Design review of the part built by this model. Coordinates are the model's own, in mm. A direction names the side the tool comes from. Give positions to 0.01 mm unless a question says otherwise; leave off trailing zeros. Loops run counter-clockwise (first coordinate to the right, second up) from the corner with the lowest first, then second, coordinate; pieces in that order, holes last. Notation, with made-up numbers: (43, 9) -> (69, 9) arc R12 ccw to (69, 23) -> close; hole circle Ø11 at (36.5, -8). An arc over 180 degrees is marked (long way). Use CSV: the item, a comma, the result in double quotes. Start each with the question number.
Item 1: We need section C-C (z = 0). State the section outline as (x, y) points, plus the area to 3 significant figures.
Item 2: Clearance check with flat-ended pins moving along their axes: pin 1 (0.6 mm diameter, centred on x = 16.5, z = -1.5, fed in from -Y); pin 2 (1 mm diameter, centred on x = 7.5, y = 1, fed in from -Z); pin 3 (1 mm diameter, centred on y = 1, z = -0.5, fed in from +X). State where each tip first meets the part, or that it passes through.
Item 3: We need section D-D (x = 10.75). State the section outline as (y, z) points, plus the area to 3 significant figures.
Item 4: The part is to be moulded in two halves that separate along Z. For faces 4 (the face through (16, 0, -1.677)), 5 (the face through (13.9, 0, 0)), 6 (the face through (16, 0, 1.677)), 7 (the face through (2.03, -1.08, -4.88)), say which applies: +Z half, -Z half, draft (parallel to the pull), parting line (faces both ways), or undercut.
Item 5: Wall thickness on line 1 along X through (y, z) = (-0.75, 3.75); line 2 along X through (y, z) = (0.75, 0); line 3 along Z through (x, y) = (2.5, -3): over which ranges is each line inside the solid? List them lowest first. Write a range as from..to.
Item 6: We need section A-A (x = 15.5). State the section outline as (y, z) points, plus the area to 3 significant figures.
Item 7: For faces 1 (the face through (0, 0, 0)), 2 (the face through (16, 0, 1.177)), 3 (the face through (6.281, -0.867, -3.905)), list the 3-axis set-ups (+Z, -Z, +X, -X, +Y, -Y) from which the entire face can be reached by the end or side of a thin tool; tool diameter is ignored.
Item 8: We need section B-B (y = 0). State the section outline as (x, z) points.
Autodesk Inventor part; units mm, degrees
ref_plane "YZ Plane" through (0, 0, 0) normal (1, 0, 0) x (0, 1, 0)
ref_plane "XZ Plane" through (0, 0, 0) normal (0, 1, 0) x (-1, 0, 0)
ref_plane "XY Plane" through (0, 0, 0) normal (0, 0, 1) x (1, 0, 0)
sketch "スケッチ1" plane through (0, 0, 0) normal (0, 0, 1) x (1, 0, 0)
  line L0 (0, 0) -> (0, 5)
  line L1 (0, 5) -> (4, 5)
  line L2 (4, 5) -> (4, 4)
  line L3 (4, 4) -> (8.5, 4)
  line L4 (8.5, 4) -> (8.5, 3.5)
  line L5 (8.5, 3.5) -> (12, 3.5)
  line L6 (12, 3.5) -> (12, 2.25)
  line L7 (12, 2.25) -> (13.9, 2.25)
  line L8 (13.9, 2.25) -> (13.9, 0)
  line L9 (13.9, 0) -> (0, 0)
  dimension "d0" = 4
  dimension "d1" = 4.5
  dimension "d2" = 8
  dimension "d3" = 1.9
  dimension "d4" = 5
  dimension "d5" = 4
  dimension "d6" = 3.5
  dimension "d7" = 2.25
revolve "回転1" add sketch "スケッチ1" angle 360 about axis through (13.9, 0, 0) along (-1, 0, 0)
sketch "スケッチ2" plane through (13.9, 0, 0) normal (1, 0, 0) x (0, 0, -1)
  circle A0 centre (0, 0) radius 2.25
  line L0 (-1.6771, 1.5) -> (-1.1771, 1.5)
  line L1 (-1.1771, 1.5) -> (-1.1771, -1.5)
  line L2 (-1.1771, -1.5) -> (-1.6771, -1.5)
  line L3 (-1.6771, -1.5) -> (-1.6771, 1.5)
  line L4 (1.6771, 1.5) -> (1.1771, 1.5)
  line L5 (1.1771, 1.5) -> (1.1771, -1.5)
  line L6 (1.1771, -1.5) -> (1.6771, -1.5)
  line L7 (1.6771, -1.5) -> (1.6771, 1.5)
  point P0 (-1.1771, 0)
  point P1 (1.1771, 0)
  dimension "d9" = 3
  dimension "d10" = 0.5
extrude "押し出し1" add sketch "スケッチ2" along normal blind 4.1 contours L7 L6 L5 L4 | L0 L1 L2 L3
properties part number "MJ-14"
Results found:
1,outline,"(0, -5) -> (4, -5) -> (4, -4) -> (8.5, -4) -> (8.5, -3.5) -> (12, -3.5) -> (12, -2.25) -> (13.9, -2.25) -> (13.9, 2.25) -> (12, 2.25) -> (12, 3.5) -> (8.5, 3.5) -> (8.5, 4) -> (4, 4) -> (4, 5) -> (0, 5) -> close"
1,area,"109 mm²"
2,pin 1,"y = -1.5"
2,pin 2,"z = -3.97"
2,pin 3,"x = 13.9"
3,outline,"circle Ø7 at (0, 0)"
3,area,"38.5 mm²"
4,face 4,"-Z half"
4,face 5,"undercut"
4,face 6,"+Z half"
4,face 7,"parting line"
5,line 1,"0..8.5"
5,line 2,"0..13.9"
5,line 3,"-4..4"
6,outline,"(-1.5, -1.68) -> (1.5, -1.68) -> (1.5, -1.18) -> (-1.5, -1.18) -> close; (-1.5, 1.18) -> (1.5, 1.18) -> (1.5, 1.68) -> (-1.5, 1.68) -> close"
6,area,"3.00 mm²"
7,face 1,"+Z, -Z, -X, +Y, -Y"
7,face 2,"+X, +Y, -Y"
7,face 3,"+X"
8,outline,"(0, -5) -> (4, -5) -> (4, -4) -> (8.5, -4) -> (8.5, -3.5) -> (12, -3.5) -> (12, -2.25) -> (13.9, -2.25) -> (13.9, -1.68) -> (18, -1.68) -> (18, -1.18) -> (13.9, -1.18) -> (13.9, 1.18) -> (18, 1.18) -> (18, 1.68) -> (13.9, 1.68) -> (13.9, 2.25) -> (12, 2.25) -> (12, 3.5) -> (8.5, 3.5) -> (8.5, 4) -> (4, 4) -> (4, 5) -> (0, 5) -> close"
